from build123d import *

# Parameters (mm, degrees)
RESSALTO_EXTRUS_O1_DEPTH = 6


with BuildPart() as part:
    # Esboço1 → Ressalto-extrusão1 (new body)
    with BuildSketch(Plane(origin=(0, 0, 0), x_dir=(1, 0, 0), z_dir=(0, 1, 0))):
        Polygon((-80, 80), (-74, 80), (-74, 60), (-80, 60), (-80, 40), (-74, 40), (-74, 20), (-80, 20), (-80, 0), (-60, 0), (-60, -6), (-50, -6), (-50, 0), (-30, 0), (-30, -6), (-20, -6), (-20, 0), (0, 0), (0, 20), (-6, 20), (-6, 40), (0, 40), (0, 60), (-6, 60), (-6, 80), (0, 80), (0, 106), (-30, 106), (-30, 100), (-50, 100), (-50, 106), (-80, 106), align=None)
    extrude(amount=RESSALTO_EXTRUS_O1_DEPTH)


solid = part.part
Check sheet for the modelled part. Datum: model origin and axes. Units: mm. A direction names the side the tool comes from. Coordinates: 2 decimals unless noted, no trailing zeros. Write each loop counter-clockwise with the first axis right and the second up, starting at its lowest first coordinate (ties: lowest second). Pieces come first, ordered by that corner, then holes. Notation, with made-up numbers: M 80.25,85.25 L 89.25,85.25 A24 ccw 89.25,100.25 Z; hole C 12.5,5 d9. An arc over 180 degrees is marked long. Answer as CSV lines item,"result".
Q1. Cross-section at B-B (x = -16). Record the boundary of the cut face in (y, z), then the cut area to 3 significant figures.
Check result:
outline,"M 0,-106 L 6,-106 L 6,0 L 0,0 Z"
area,"636 mm^2"
Q2. Cross-section at C-C (z = -76.5). Record the boundary of the cut face in (x, y).
Check result:
outline,"M -74,0 L -6,0 L -6,6 L -74,6 Z"
Q3. Set-up check for faces 1 (the face through (-74, 3, -70)), 2 (the face through (-20, 3, 3)), 3 (the face through (-40, 3, 0)): record each of +Z, -Z, +X, -X, +Y, -Y from which the full face is reachable in a straight line by a thin tool's end or side.
Check result:
face 1,"-X, +Y, -Y"
face 2,"+Z, +X, +Y, -Y"
face 3,"+Z, +Y, -Y"
Q4. Go/stop test with flat-tipped pins: pin 1 (1.8 mm diameter, centred on y = 2.5, z = 4, fed in from -X); pin 2 (1.8 mm diameter, centred on x = -11.5, y = 4.5, fed in from +Z); pin 3 (1.8 mm diameter, centred on y = 3, z = -66.5, fed in from +X); pin 4 (12 mm diameter, centred on x = -60, z = -59, fed in from -Y). Record where each tip stops, or that it passes through.
Check result:
pin 1,"x = -60"
pin 2,"z = 0"
pin 3,"x = -6"
pin 4,"y = 0"
Q5. Mould release check, pull along X, two halves, no side actions. Record for faces 4 (the face through (-74, 3, -30)), 5 (the face through (-41, 0, -51)), 6 (the face through (-30, 3, -103)): released by +X, released by -X, zero draft, split by the parting line, or undercut.
Check result:
face 4,"released by -X"
face 5,"zero draft"
face 6,"undercut"
Q6. Material ranges on probe 1 along X at (y, z) = (3.1, -100.5); probe 2 along X at (y, z) = (3.4, 0.5); probe 3 along Z at (x, y) = (-40, 5.4), recorded low to high. Write a range as from..to.
Check result:
probe 1,"-80..-50, -30..0"
probe 2,"-60..-50, -30..-20"
probe 3,"-100..0"
